Can you work these out from the model? Positions are in its coordinate system, mm. A direction names the side the tool comes from. Give positions to 0.01 mm unless a question says otherwise; leave off trailing zeros. Write each loop counter-clockwise with the first axis right and the second up, starting at its lowest first coordinate (ties: lowest second). Pieces come first, ordered by that corner, then holes. Notation, with made-up numbers: (-8, 75) - (20, 75) arc R30 cw to (20, 111) - close; hole circle Ø11 at (49.5, 1). An arc over 180 degrees is marked (long way). Use a Markdown table: item, result. Add a question column.
```python
from build123d import *
from OCP.BRepFilletAPI import BRepFilletAPI_MakeChamfer

# Parameters (mm, degrees)
BOSS_EXTRUDE1_DEPTH        = 9.525
BOSS_EXTRUDE2_DEPTH        = 12.7
CUT_EXTRUDE1_DEPTH         = 5.08
F_10_32_TAPPED_HOLE1_D     = 4.0386
F_10_32_TAPPED_HOLE1_DEPTH = 4.445
F_10_CLEARANCE_HOLE1_D     = 4.9784
F_10_CLEARANCE_HOLE1_DEPTH = 14.604
CUT_EXTRUDE2_DEPTH         = 1.778
F_10_CLEARANCE_HOLE2_D     = 4.9784
F_10_CLEARANCE_HOLE2_DEPTH = 8.127
F_10_32_TAPPED_HOLE2_D     = 4.0386
CHAMFER1_SIZE              = 1.27
CHAMFER1_SIZE2             = 1.568319389


with BuildPart() as part:
    # Sketch1 → Boss-Extrude1 (new, symmetric)
    with BuildSketch(Plane(origin=(0, 0, 0), x_dir=(1, 0, 0), z_dir=(0, 1, 0))):
        with BuildLine():
            Line((0, -6.35), (-19.05, -6.35))
            ThreePointArc((-19.05, -6.35), (-25.4, 0), (-19.05, 6.35))
            Line((-19.05, 6.35), (0, 6.35))
            Line((0, 6.35), (0, -6.35))
        make_face()
    extrude(amount=BOSS_EXTRUDE1_DEPTH, both=True)

    # Sketch2 → Boss-Extrude2 (add)
    with BuildSketch(Plane.XY.offset(6.35)):
        with BuildLine():
            Line((0, 9.525), (6.35, 9.525))
            ThreePointArc((6.35, 9.525), (15.875, 0), (6.35, -9.525))
            Line((6.35, -9.525), (0, -9.525))
            ThreePointArc((0, -9.525), (-9.525, 0), (0, 9.525))
        make_face()
    extrude(amount=-BOSS_EXTRUDE2_DEPTH)

    # Sketch3 → Cut-Extrude1 (cut, symmetric)
    with BuildSketch(Plane(origin=(0, 0, 0), x_dir=(1, 0, 0), z_dir=(0, 1, 0))):
        with BuildLine():
            Line((-12.526499966, 6.35), (-19.05, 6.35))
            ThreePointArc((-19.05, 6.35), (-25.4, 0), (-19.05, -6.35))
            Line((-19.05, -6.35), (-12.526499966, -6.35))
            Line((-12.526499966, -6.35), (-12.526499966, 6.35))
        make_face()
    extrude(amount=CUT_EXTRUDE1_DEPTH, both=True, mode=Mode.SUBTRACT)

    # #10-32 Tapped Hole1
    with Locations(Plane(origin=(0, -5.08, 0), x_dir=(1, 0, 0), z_dir=(0, 1, 0))):
        with Locations((-19.05, 0)):
            Hole(F_10_32_TAPPED_HOLE1_D / 2, depth=F_10_32_TAPPED_HOLE1_DEPTH)

    # #10 Clearance Hole1
    with Locations(Plane(origin=(0, 9.525, 0), x_dir=(1, 0, 0), z_dir=(0, 1, 0))):
        with Locations((-19.05, 0)):
            Hole(F_10_CLEARANCE_HOLE1_D / 2, depth=F_10_CLEARANCE_HOLE1_DEPTH)

    # Sketch9 → Cut-Extrude2 (cut, symmetric)
    with BuildSketch(Plane.XY):
        with BuildLine():
            Line((-5.976257023, 0), (-8.528473081, -9.525))
            Line((-8.528473081, -9.525), (6.35, -9.525))
            ThreePointArc((6.35, -9.525), (15.875, 0), (6.35, 9.525))
            Line((6.35, 9.525), (-8.528473081, 9.525))
            Line((-8.528473081, 9.525), (-5.976257023, 0))
        make_face()
    extrude(amount=CUT_EXTRUDE2_DEPTH, both=True, mode=Mode.SUBTRACT)

    # #10 Clearance Hole2
    with Locations(Plane(origin=(0, 0, -6.35), x_dir=(-1, 0, 0), z_dir=(0, 0, -1))):
        with Locations((-6.35, 0)):
            Hole(F_10_CLEARANCE_HOLE2_D / 2, depth=F_10_CLEARANCE_HOLE2_DEPTH)

    # #10-32 Tapped Hole2 (through all)
    with Locations(Plane(origin=(0, 0, 1.778), x_dir=(-1, 0, 0), z_dir=(0, 0, -1))):
        with Locations((-6.35, 0)):
            Hole(F_10_32_TAPPED_HOLE2_D / 2)

    # Chamfer1: one chamfer whose edges measure the first distance from different faces: ONE call of the kernel's chamfer builder (chamfer() names one face for all edges)
    chamfer1_edges_1 = [part.edges().sort_by_distance(p)[0] for p in [
        (-1.08923654, -9.525, -1.778),
    ]]
    chamfer1_side_1 = [part.faces().sort_by_distance(p)[0] for p in [
        (-9.756442015, -9.525, 0),
    ]]
    chamfer1_edges_2 = [part.edges().sort_by_distance(p)[0] for p in [
        (15.875, 0, -1.778),
    ]]
    chamfer1_side_2 = [part.faces().sort_by_distance(p)[0] for p in [
        (15.875, 0, -4.064),
    ]]
    chamfer1_edges_3 = [part.edges().sort_by_distance(p)[0] for p in [
        (-1.08923654, 9.525, -1.778),
    ]]
    chamfer1_side_3 = [part.faces().sort_by_distance(p)[0] for p in [
        (-9.559168107, 9.525, 0),
    ]]
    chamfer1_edges_4 = [part.edges().sort_by_distance(p)[0] for p in [
        (-1.08923654, -9.525, 1.778),
        (15.875, 0, 1.778),
        (-1.08923654, 9.525, 1.778),
    ]]
    chamfer1_side_4 = [part.faces().sort_by_distance(p)[0] for p in [
        (3.285858214, 0, 1.778),
    ]]
    chamfer1 = BRepFilletAPI_MakeChamfer(part.part.solid().wrapped)
    for e in chamfer1_edges_1:
        chamfer1.Add(CHAMFER1_SIZE, CHAMFER1_SIZE2, e.wrapped, chamfer1_side_1[0].wrapped)  # the first distance lies on this face
    for e in chamfer1_edges_2:
        chamfer1.Add(CHAMFER1_SIZE, CHAMFER1_SIZE2, e.wrapped, chamfer1_side_2[0].wrapped)  # the first distance lies on this face
    for e in chamfer1_edges_3:
        chamfer1.Add(CHAMFER1_SIZE, CHAMFER1_SIZE2, e.wrapped, chamfer1_side_3[0].wrapped)  # the first distance lies on this face
    for e in chamfer1_edges_4:
        chamfer1.Add(CHAMFER1_SIZE, CHAMFER1_SIZE2, e.wrapped, chamfer1_side_4[0].wrapped)  # the first distance lies on this face
    add(Compound.cast(chamfer1.Shape()), mode=Mode.REPLACE)


solid = part.part
```
Q1. If I drill on probe 1 along Z at (x, y) = (6, -3.75); probe 2 along Z at (x, y) = (5.5, 8.25); probe 3 along Y at (x, z) = (-22, 1.5) (3 decimals), over which ranges is the centre line in solid material (lowest first)? Write a range as [from, to].
Q2. Suppose I cut it at C-C (x = -0.5). Please give me the cut outline in (y, z) (3 decimals), and give its area (3 significant figures).
Q3. If we mould it in two halves opening along Z, with no side actions, what happens to faces 6 (the flat face through (-1.193, -8.899, 2.573)), 7 (the cylindrical face through (15.873, 0.209, 4.869)), 8 (the cylindrical face through (-25.4, 7.3, 0.1)), 9 (the flat face through (-1, 0, 6.35))? For each: released by +Z, released by -Z, zero draft, split by the parting line, or undercut.
Q4. Suppose I cut it at A-A (x = -15). Please give me the cut outline in (y, z) (3 decimals), and give its area (3 significant figures).
Q5. On a 3-axis mill with a long thin cutter (end or side, diameter ignored), from which of +Z, -Z, +X, -X, +Y, -Y can I reach the whole of each face in a straight line? I mean faces 1 (the conical face through (14.7, -0.2, 1.9)), 2 (the flat face through (-16, 5.08, 0)), 3 (the cylindrical face through (-16.563, 7.271, -0.109)), 4 (the flat face through (-7.27, 4.83, 0.19)), 5 (the flat face through (-7.234, -4.696, 0.194)). Say none if no direction works.
Q6. I'm going to push flat-ended pins straight in: P1, Ø3.5, axis at x = 6.35, y = 0, coming from the +Z side; P2, Ø1, axis at y = -3.5, z = 1, coming from the +X side. Where does each tip first touch, or does it pass through?
Q7. Suppose I cut it at B-B (z = 0). Please give me the cut outline in (x, y) (1 decimal), and give its area (3 significant figures).
Derived:
| question | item | result |
|---|---|---|
| 1 | probe 1 | [-6.35, -1.78], [1.78, 6.35] |
| 1 | probe 2 | [-6.35, -2.02], [1.78, 6.35] |
| 1 | probe 3 | [-9.525, -5.08], [5.08, 9.525] |
| 2 | outline | (-9.525, -6.35) - (9.525, -6.35) - (9.525, -3.048) - (7.957, -1.778) - (-7.957, -1.778) - (-9.525, -3.048) - close; (-9.525, 3.346) - (-8.255, 1.778) - (8.255, 1.778) - (9.525, 3.346) - (9.525, 6.35) - (-9.525, 6.35) - close |
| 2 | area | 170 mm² |
| 3 | face 6 | undercut |
| 3 | face 7 | zero draft |
| 3 | face 8 | split by the parting line |
| 3 | face 9 | released by +Z |
| 4 | outline | (-9.525, -6.35) - (-5.08, -6.35) - (-5.08, 6.35) - (-9.525, 6.35) - close; (5.08, -6.35) - (9.525, -6.35) - (9.525, 6.35) - (5.08, 6.35) - close |
| 4 | area | 113 mm² |
| 5 | face 1 | +X |
| 5 | face 2 | +Z, -Z, -X |
| 5 | face 3 | +Y |
| 5 | face 4 | +X, +Y |
| 5 | face 5 | +X, -Y |
| 6 | P1 | through |
| 6 | P2 | x = -6.78 |
| 7 | outline | (-25.4, -9.5) - (-21.1, -9.5) - (-21.1, -5.1) - (-25.4, -5.1) - close; (-25.4, 5.1) - (-21.5, 5.1) - (-21.5, 9.5) - (-25.4, 9.5) - close; (-17, -9.5) - (-8.5, -9.5) - (-6, 0) - (-8.5, 9.5) - (-16.6, 9.5) - (-16.6, 5.1) - (-12.5, 5.1) - (-12.5, -5.1) - (-17, -5.1) - close |
| 7 | area | 175 mm² |
